Source: CAD feature listing. Evaluate the final solid. Frame: model axes, mm. Face numbers are marked on the shaded views. A direction names the side the tool comes from. Round coordinates to 2 decimals unless told otherwise and drop trailing zeros. Order: outer loops, then holes, each group sorted by start corner. A loop starts at its lowest first (then second) coordinate and runs counter-clockwise, first axis right, second up. Notation, with made-up numbers: (30, -38.5) - (49, -38.5) arc R14 cw to (49, -26.5) - close; hole circle Ø7 at (16.5, 49). An arc over 180 degrees is marked (long way). Use one line per item in the form item = value. Start each with the question number.
Q1. Cut plane C-C, the plane x = -17.25. Return the cut outline in (y, z).
Q2. Ray query, line 1 (Y direction, x = 14.75, z = -3.15); line 2 (Y direction, x = -15.5, z = -3.75); line 3 (X direction, y = -7.5, z = -1). Return the intervals inside material, ascending. Write a range as [from, to].
Q3. Pin query (flat end, axial travel): pin 1 Ø0.5 at (x, y) = (15, -11) entering from -Z; pin 2 Ø6 at (x, y) = (-1, 1.5) entering from -Z. Return the tip coordinate at first contact, or that it passes through.
Q4. Cut plane B-B, the plane y = -2. Return the cut outline in (x, z).
Q5. Cut plane D-D, the plane z = -1. Return the cut outline in (x, y), and give its area (3 significant figures).
Q6. Cut plane A-A, the plane x = 14.75. Return the cut outline in (y, z), and give its area (3 significant figures).
Q7. Set-up query: the marked faces 4 and 5. Return all of +Z, -Z, +X, -X, +Y, -Y with unobstructed straight access to the full face (end or side cutting, diameter ignored); none if empty.
Q8. Draft query along X for the marked faces 1, 2 and 3. Return one class per face: released by +X, released by -X, zero draft, split by the parting line, or undercut.
from build123d import *

# Parameters (mm, degrees)
SKETCH1_W           = 36
SKETCH1_H           = 26
SKETCH1_W_2         = 30
SKETCH1_H_2         = 20
EXTRUDE_THIN1_DEPTH = 5.5
CUT_EXTRUDE1_REACH  = 40.668
SKETCH1_4_W         = 36
SKETCH1_4_H         = 26
SKETCH1_4_W_2       = 30
SKETCH1_4_H_2       = 20
BOSS_EXTRUDE3_DEPTH = 2
SKETCH4_R           = 0.9
CUT_EXTRUDE4_DEPTH  = 5
CUT_EXTRUDE5_REACH  = 40.668
SKETCH5_R           = 0.5


with BuildPart() as part:
    # Sketch1 → Extrude-Thin1 (new body)
    with BuildSketch(Plane.XY):
        with Locations((-1.25, 0)):
            Rectangle(SKETCH1_W, SKETCH1_H)
        with Locations((-1.25, 0)):
            Rectangle(SKETCH1_W_2, SKETCH1_H_2, mode=Mode.SUBTRACT)
    extrude(amount=-EXTRUDE_THIN1_DEPTH)

    # Sketch2 → Cut-Extrude1 (cut, up to next)
    with BuildSketch(Plane(origin=(16.75, 0, 0), x_dir=(0, 0, -1), z_dir=(1, 0, 0)), mode=Mode.PRIVATE) as cut_extrude1_sk1:
        Polygon((4.5, -3.9), (4.5, 3.9), (3.1, 3.9), (2.3, 2.6), (2.3, 0), (2.3, -2.6), (3.1, -3.9), align=None)
    cut_extrude1_tool1 = extrude(cut_extrude1_sk1.sketch, amount=-CUT_EXTRUDE1_REACH, mode=Mode.PRIVATE) & part.part
    add(cut_extrude1_tool1.solids().sort_by_distance((16.75, 0, -3.453763))[0], mode=Mode.SUBTRACT)

    # Sketch1<4> → Boss-Extrude3 (add)
    # profile 1 of 2: a face of its own
    with BuildSketch(Plane.XY):
        with Locations((-1.25, 0)):
            Rectangle(SKETCH1_4_W, SKETCH1_4_H)
        with Locations((-1.25, 0)):
            Rectangle(SKETCH1_4_W_2, SKETCH1_4_H_2, mode=Mode.SUBTRACT)
    # profile 2 of 2: a face of its own
    with BuildSketch(Plane.XY):
        with Locations((-1.25, 0)):
            Rectangle(SKETCH1_4_W_2, SKETCH1_4_H_2)
    extrude(amount=BOSS_EXTRUDE3_DEPTH)

    # Sketch4 → Cut-Extrude4 (cut)
    with BuildSketch(Plane(origin=(0, 0, -5.5), x_dir=(-1, 0, 0), z_dir=(0, 0, -1))):
        with Locations((-14.75, 11)):
            Circle(SKETCH4_R)
        with Locations((17.25, 11)):
            Circle(SKETCH4_R)
        with Locations((17.25, -11)):
            Circle(SKETCH4_R)
        with Locations((-14.75, -11)):
            Circle(SKETCH4_R)
    extrude(amount=-CUT_EXTRUDE4_DEPTH, mode=Mode.SUBTRACT)

    # Sketch5 → Cut-Extrude5 (cut, up to next)
    with BuildSketch(Plane.ZY.offset(19.25), mode=Mode.PRIVATE) as cut_extrude5_sk1:
        with Locations(Location((-2.5, 4.2, 0), (0, 0, 270))):
            Circle(SKETCH5_R)
    cut_extrude5_tool1 = extrude(cut_extrude5_sk1.sketch, amount=-CUT_EXTRUDE5_REACH, mode=Mode.PRIVATE) & part.part
    # Sketch5 → Cut-Extrude5 (cut, up to next)
    with BuildSketch(Plane.ZY.offset(19.25), mode=Mode.PRIVATE) as cut_extrude5_sk2:
        with Locations(Location((-2.5, -4.2, 0), (0, 0, 270))):
            Circle(SKETCH5_R)
    cut_extrude5_tool2 = extrude(cut_extrude5_sk2.sketch, amount=-CUT_EXTRUDE5_REACH, mode=Mode.PRIVATE) & part.part
    add(cut_extrude5_tool1.solids().sort_by_distance((-19.25, 4.2, -2.5))[0], mode=Mode.SUBTRACT)
    add(cut_extrude5_tool2.solids().sort_by_distance((-19.25, -4.2, -2.5))[0], mode=Mode.SUBTRACT)


solid = part.part
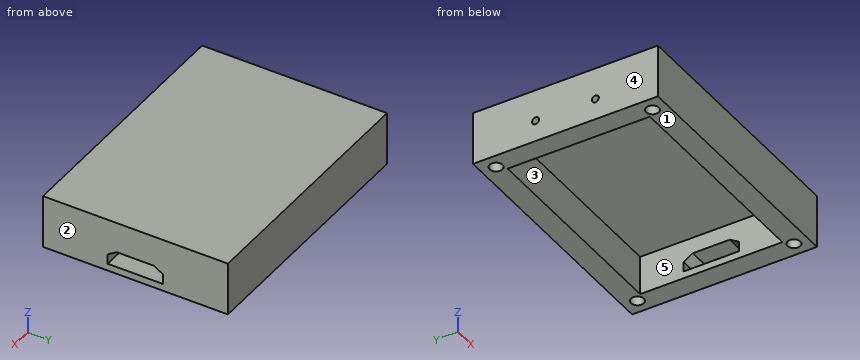
Completed:
q1.outline = (-13, -5.5) - (-11.9, -5.5) - (-11.9, -0.5) - (-10.1, -0.5) - (-10.1, -5.5) - (10.1, -5.5) - (10.1, -0.5) - (11.9, -0.5) - (11.9, -5.5) - (13, -5.5) - (13, 2) - (-13, 2) - close; hole circle Ø1 at (-4.2, -2.5); hole circle Ø1 at (4.2, -2.5)
q2.line_1 = [-13, -11.9], [-10.1, -3.9], [3.9, 10.1], [11.9, 13]
q2.line_2 = [-13, -10], [10, 13]
q2.line_3 = [-19.25, -16.25], [13.75, 16.75]
q3.pin_1 = -0.5
q3.pin_2 = 0
q4.outline = (-19.25, -5.5) - (-16.25, -5.5) - (-16.25, 0) - (13.75, 0) - (13.75, -2.3) - (16.75, -2.3) - (16.75, 2) - (-19.25, 2) - close; (13.75, -5.5) - (16.75, -5.5) - (16.75, -4.5) - (13.75, -4.5) - close
q5.outline = (-19.25, -13) - (16.75, -13) - (16.75, 13) - (-19.25, 13) - close; hole circle Ø1.8 at (-17.25, -11); hole circle Ø1.8 at (-17.25, 11); hole (-16.25, -10) - (13.75, -10) - (13.75, 10) - (-16.25, 10) - close; hole circle Ø1.8 at (14.75, -11); hole circle Ø1.8 at (14.75, 11)
q5.area = 326 mm2
q6.outline = (-13, -5.5) - (-11.9, -5.5) - (-11.9, -0.5) - (-10.1, -0.5) - (-10.1, -5.5) - (10.1, -5.5) - (10.1, -0.5) - (11.9, -0.5) - (11.9, -5.5) - (13, -5.5) - (13, 2) - (-13, 2) - close; hole (-3.9, -4.5) - (3.9, -4.5) - (3.9, -3.1) - (2.6, -2.3) - (-2.6, -2.3) - (-3.9, -3.1) - close
q6.area = 161 mm2
q7.face_4 = +Z, -Z, -X, +Y, -Y
q7.face_5 = -Z
q8.face_1 = zero draft
q8.face_2 = released by +X
q8.face_3 = undercut
